Model file for the job. Use its own axes, mm. Give positions to 0.01 mm unless a question says otherwise; leave off trailing zeros. Loops run counter-clockwise (first coordinate to the right, second up) from the corner with the lowest first, then second, coordinate; pieces in that order, holes last. Notation, with made-up numbers: M -14.75,61.25 L 15.25,61.25 A22 cw 15.25,75.25 Z; hole C -36.5,-17.5 d8. An arc over 180 degrees is marked long. Use CSV: the item, a comma, the result in double quotes. Start each with the question number.
(1) Slice it at A-A on y = 83. List the corners of the cut face in (x, z).
(2) Two-plate mould, pull along Y, no slides. Class faces 1 (the face through (7.195, 84.487, 2.958)), 2 (the face through (64, 0, 3)), 3 (the face through (130, 44, 3)), 4 (the face through (124.11, 84.01, 2.96)): pulls with the +Y half, pulls with the -Y half, needs draft (parallel to the pull), parting line crosses it, or undercut.
(3) Slice it at B-B on x = 123. List the corners of the cut face in (y, z).
(4) Wall check: line 1 along X through (y, z) = (75.1, 3.5); line 2 along X through (y, z) = (83, 2.5). Give the ranges that are in metal, low to high. Write a range as from..to.
```python
from build123d import *

# Parameters (mm, degrees)
SKETCH1_W             = 130
SKETCH1_H             = 90
BOSS_EXTRUDE1_DEPTH   = 6
F_3_0MM_DOWEL_HOLE1_D = 3
F_2_0MM_DOWEL_HOLE1_D = 2


with BuildPart() as part:
    # Sketch1 → Boss-Extrude1 (new body)
    with BuildSketch(Plane.XY):
        with Locations((65, 45)):
            Rectangle(SKETCH1_W, SKETCH1_H)
    extrude(amount=BOSS_EXTRUDE1_DEPTH)

    # Ø3.0mm Dowel Hole1 (through all)
    with Locations(Plane.XY.offset(6)):
        with Locations((123, 83), (123, 7), (7, 7), (7, 83)):
            Hole(F_3_0MM_DOWEL_HOLE1_D / 2)

    # Ø2.0mm Dowel Hole1 (through all)
    with Locations(Plane(origin=(0, 0, 0), x_dir=(-1, 0, 0), z_dir=(0, 0, -1))):
        with Locations((-114, 75.1), (-114, 15.1), (-15.82, 14.89), (-15.82, 75)):
            Hole(F_2_0MM_DOWEL_HOLE1_D / 2)


solid = part.part
```
Reply:
1,outline,"M 0,0 L 5.5,0 L 5.5,6 L 0,6 Z; M 8.5,0 L 121.5,0 L 121.5,6 L 8.5,6 Z; M 124.5,0 L 130,0 L 130,6 L 124.5,6 Z"
2,face 1,"undercut"
2,face 2,"pulls with the -Y half"
2,face 3,"needs draft"
2,face 4,"undercut"
3,outline,"M 0,0 L 5.5,0 L 5.5,6 L 0,6 Z; M 8.5,0 L 81.5,0 L 81.5,6 L 8.5,6 Z; M 84.5,0 L 90,0 L 90,6 L 84.5,6 Z"
4,line 1,"x = 0..14.83, 16.81..113, 115..130"
4,line 2,"x = 0..5.5, 8.5..121.5, 124.5..130"
